Answer from the drawing. Dimensions are ordinates in mm from the lowest x, y and z of the part. A direction names the side the tool comes from. Give positions to 0.01 mm unless a question says otherwise; leave off trailing zeros. Write each loop counter-clockwise with the first axis right and the second up, starting at its lowest first coordinate (ties: lowest second). Pieces come first, ordered by that corner, then holes. Notation, with made-up numbers: M 16,2 L 34,2 A5 cw 34,6 Z; hole C 76,13.25 d1. An arc over 180 degrees is marked long. Answer as a JSON object with one key per item and string values.
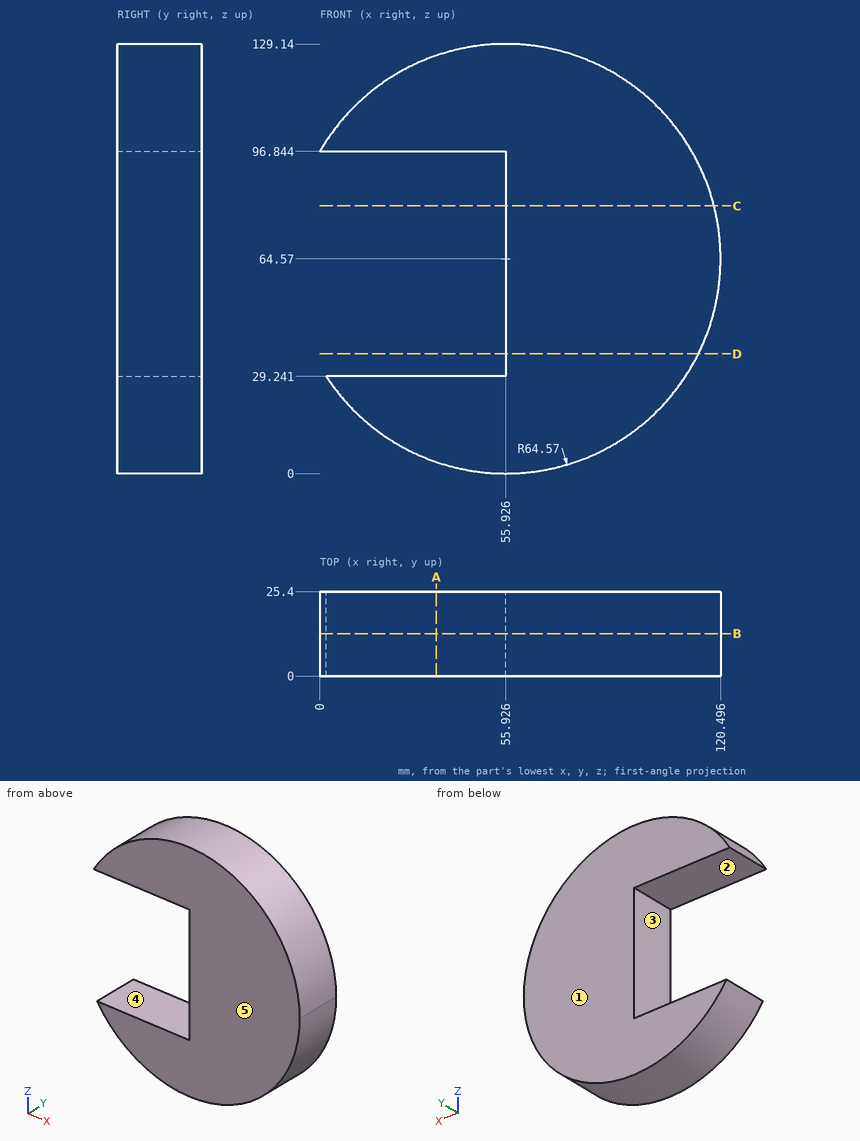
1. A cutting plane is placed at C-C, the plane z = 80.5. Give the vertices of the cut face in (x, y).
Verdict:
{"outline": "M 55.93,0 L 118.5,0 L 118.5,25.4 L 55.93,25.4 Z"}
2. A cutting plane is placed at A-A, the plane x = 35. Give the vertices of the cut face in (y, z) (1 decimal).
Verdict:
{"outline": "M 0,3.5 L 25.4,3.5 L 25.4,29.2 L 0,29.2 Z; M 0,96.8 L 25.4,96.8 L 25.4,125.7 L 0,125.7 Z"}
3. For the marked faces 1 and 2, determine the directions among +Z, -Z, +X, -X, +Y, -Y from which every point of the face is accessible in a straight line to the end or side of a thin tool.
Verdict:
{"face 1": "+Z, -Z, +X, -X, +Y", "face 2": "-X, +Y, -Y"}
4. A cutting plane is placed at B-B, the plane y = 12.75. Give the vertices of the cut face in (x, z), plus the area to 3 significant figures.
Verdict:
{"outline": "M 0,96.84 L 55.93,96.84 L 55.93,29.24 L 1.88,29.24 A64.57 ccw long Z", "area": "8,940 mm2"}
5. Flat-ended cylindrical pins translate along their axes: pin 1 (8 mm diameter, centred on y = 6, z = 76, fed in from +X); pin 2 (6 mm diameter, centred on y = 7, z = 80, fed in from -X); pin 3 (3 mm diameter, centred on y = 5.5, z = 113, fed in from +X) (1 decimal). Find the tip coordinate at first contact, or state that the pin passes through.
Verdict:
{"pin 1": "stops at x = 120.07", "pin 2": "stops at x = 55.93", "pin 3": "stops at x = 100.3"}
6. The mould has two halves that part along Z. Classify the marked faces 3, 4 and 5: released by +Z, released by -Z, zero draft, split by the parting line, or undercut.
Verdict:
{"face 3": "undercut", "face 4": "undercut", "face 5": "zero draft"}
7. A cutting plane is placed at D-D, the plane z = 36. Give the vertices of the cut face in (x, y), plus the area to 3 significant figures.
Verdict:
{"outline": "M 55.93,0 L 113.83,0 L 113.83,25.4 L 55.93,25.4 Z", "area": "1,470 mm2"}
8. Consider line 1 along Z through (x, y) = (25, 12.5) (1 decimal); line 2 along X through (y, z) = (13.5, 63.5); line 3 along Z through (x, y) = (49, 13). Determine where each line is inside the solid, lowest interval first.
Verdict:
{"line 1": "z = 7.9 to 29.2, 96.8 to 121.3", "line 2": "x = 55.93 to 120.49", "line 3": "z = 0.37 to 29.24, 96.84 to 128.77"}
